Answer from the drawing. Dimensions are ordinates in mm from the lowest x, y and z of the part. A direction names the side the tool comes from. Coordinates: 2 decimals unless noted, no trailing zeros. Write each loop counter-clockwise with the first axis right and the second up, starting at its lowest first coordinate (ties: lowest second). Pieces come first, ordered by that corner, then holes. Notation, with made-up numbers: (-18.75, 89) -> (26.25, 89) arc R21 ccw to (26.25, 110) -> close; hole circle Ø11 at (12.5, -22). An arc over 180 degrees is marked (long way). One line per item, written item: value. Start each with the question number.
1. Consider line 1 along X through (y, z) = (0.85, 3.3); line 2 along X through (y, z) = (1.25, 41.5); line 3 along Y through (x, z) = (27, 16.5). Determine where each line is inside the solid, lowest interval first.
2. Find section C-C, the plane z = 3.3. Write down the section's boundary in (x, y), and give its area (3 significant figures).
3. Given P1, Ø5, axis at x = 3.8, z = 3.3, coming from the -Y side; P2, Ø2, axis at y = 4.5, z = 34.5, coming from the -X side; P3, Ø4, axis at x = 41, z = 40.5, coming from the +Y side; P4, Ø2, axis at y = 4, z = 35, coming from the +X side, each flat-ended and moving along its own axis, determine where each tip first touches the part or whether it passes through.
4. Find section D-D, the plane y = 5.5. Write down the section's boundary in (x, z).
5. Find section A-A, the plane z = 40.5. Write down the section's boundary in (x, y), and give its area (3 significant figures).
6. Find section B-B, the plane x = 41. Write down the section's boundary in (y, z), and give its area (3 significant figures).
7. For the marked faces 1, 2 and 3, determine the directions among +Z, -Z, +X, -X, +Y, -Y from which every point of the face is accessible in a straight line to the end or side of a thin tool.
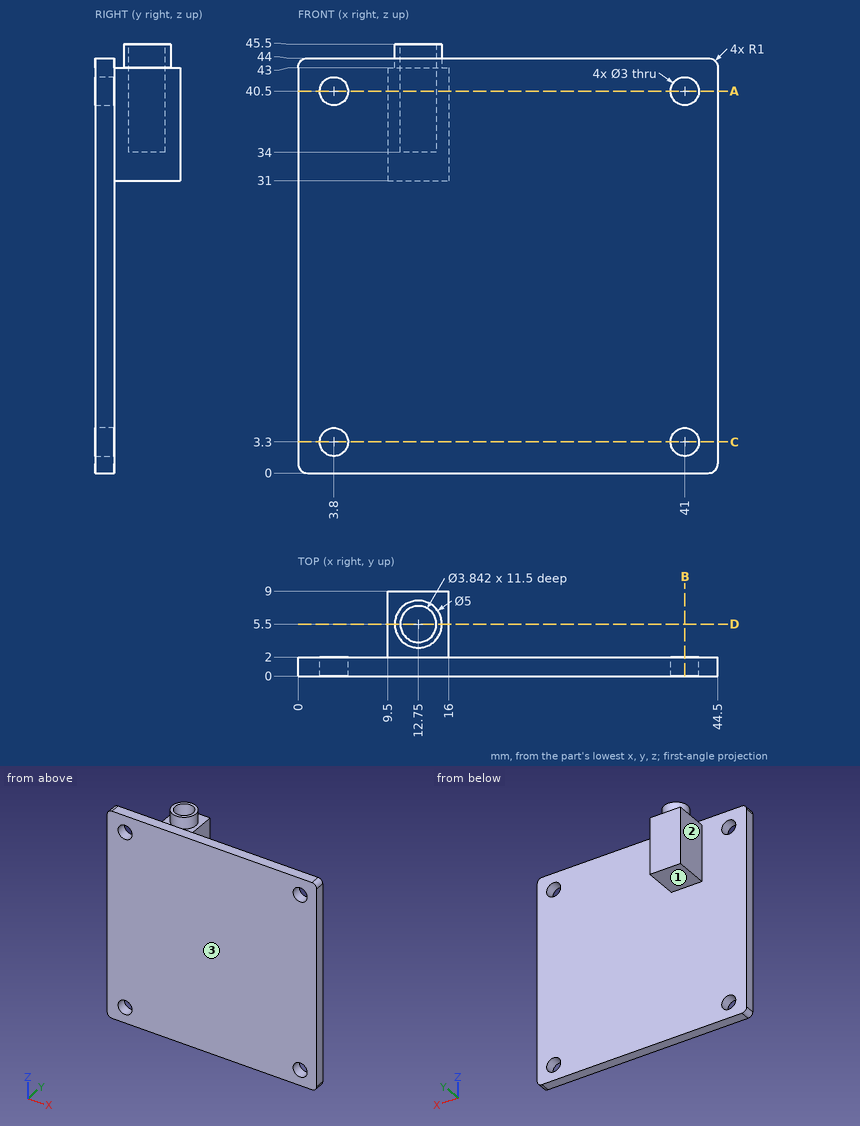
Answer block:
1. line 1: x = 0 to 2.3, 5.3 to 39.5, 42.5 to 44.5
1. line 2: x = 0 to 2.68, 4.92 to 39.88, 42.12 to 44.5
1. line 3: y = 0 to 2
2. outline: (0, 0) -> (2.3, 0) -> (2.3, 2) -> (0, 2) -> close; (5.3, 0) -> (39.5, 0) -> (39.5, 2) -> (5.3, 2) -> close; (42.5, 0) -> (44.5, 0) -> (44.5, 2) -> (42.5, 2) -> close
2. area: 77.0 mm2
3. P1: stops at y = 0
3. P2: stops at x = 9.5
3. P3: stops at y = 2
3. P4: stops at x = 16
4. outline: (9.5, 31) -> (16, 31) -> (16, 43) -> (15.25, 43) -> (15.25, 45.5) -> (14.67, 45.5) -> (14.67, 34) -> (10.83, 34) -> (10.83, 45.5) -> (10.25, 45.5) -> (10.25, 43) -> (9.5, 43) -> close
5. outline: (0, 0) -> (2.3, 0) -> (2.3, 2) -> (0, 2) -> close; (5.3, 0) -> (39.5, 0) -> (39.5, 2) -> (16, 2) -> (16, 9) -> (9.5, 9) -> (9.5, 2) -> (5.3, 2) -> close; (42.5, 0) -> (44.5, 0) -> (44.5, 2) -> (42.5, 2) -> close; hole circle Ø3.84 at (12.75, 5.5)
5. area: 111 mm2
6. outline: (0, 0) -> (2, 0) -> (2, 1.8) -> (0, 1.8) -> close; (0, 4.8) -> (2, 4.8) -> (2, 39) -> (0, 39) -> close; (0, 42) -> (2, 42) -> (2, 44) -> (0, 44) -> close
6. area: 76.0 mm2
7. face 1: -Z, +X, -X, +Y
7. face 2: +Z, -Z, -X, +Y
7. face 3: +Z, -Z, +X, -X, -Y
